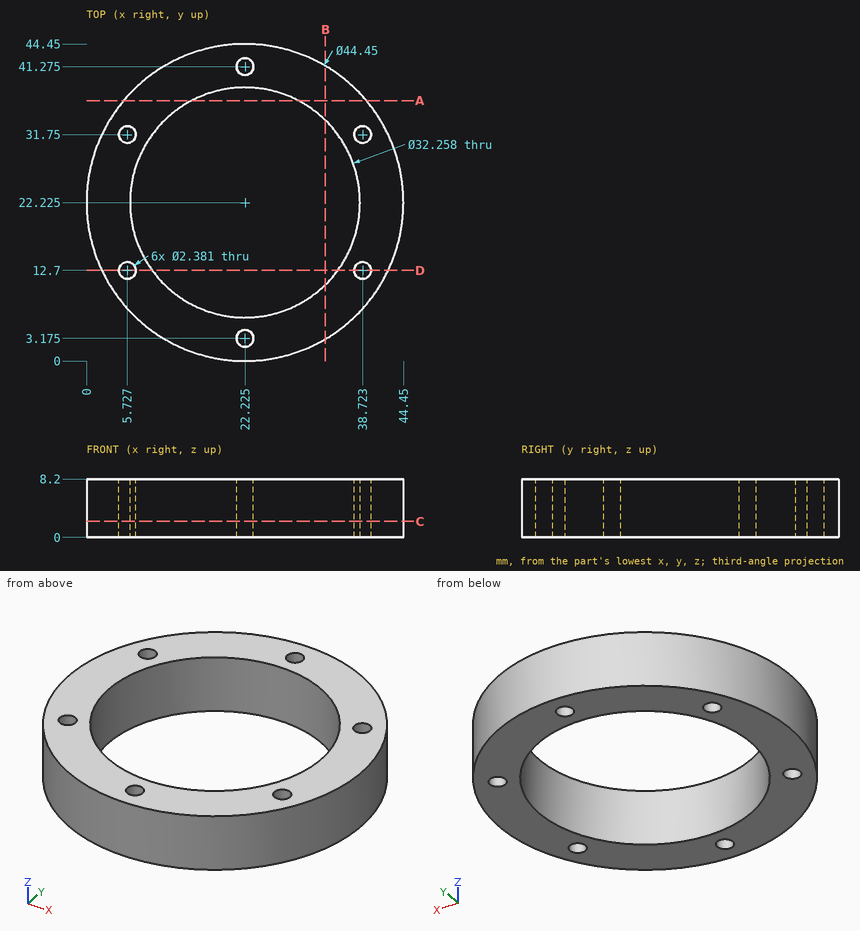
Study the drawing (mm; zero at the part's minimum x, y, z) and answer. Round coordinates to 2 decimals unless told otherwise and drop trailing zeros. Write each loop counter-clockwise with the first axis right and the second up, starting at its lowest first coordinate (ties: lowest second). Pieces come first, ordered by that corner, then holes. Notation, with made-up numbers: (35, 3.5) -> (89, 3.5) arc R25 ccw to (89, 30.5) -> close; hole circle Ø6 at (-32.5, 49.25). An arc over 180 degrees is marked (long way). Write each question's results on one line, items separated by ' | '.
Item 1: A cutting plane is placed at B-B, the plane x = 33.5. Determine the outline of the cut face in (y, z).
Result set:
outline: (3.07, 0) -> (10.69, 0) -> (10.69, 8.2) -> (3.07, 8.2) -> close; (33.76, 0) -> (41.38, 0) -> (41.38, 8.2) -> (33.76, 8.2) -> close
Item 2: Find the intervals of material crossed by line 1 along Y through (x, z) = (39, 6.75) (1 decimal); line 2 along X through (y, z) = (12.7, 5.5) (1 decimal); line 3 along Y through (x, z) = (18.5, 1.5) (1 decimal), in increasing order. Write a range as [from, to].
Result set:
line 1: [7.6, 11.5], [13.9, 30.6], [32.9, 36.8] | line 2: [2.1, 4.5], [6.9, 9.2], [35.2, 37.5], [39.9, 42.3] | line 3: [0.3, 6.5], [37.9, 44.1]
Item 3: A cutting plane is placed at D-D, the plane y = 12.7. Determine the outline of the cut face in (x, z) (1 decimal).
Result set:
outline: (2.1, 0) -> (4.5, 0) -> (4.5, 8.2) -> (2.1, 8.2) -> close; (6.9, 0) -> (9.2, 0) -> (9.2, 8.2) -> (6.9, 8.2) -> close; (35.2, 0) -> (37.5, 0) -> (37.5, 8.2) -> (35.2, 8.2) -> close; (39.9, 0) -> (42.3, 0) -> (42.3, 8.2) -> (39.9, 8.2) -> close
Item 4: Flat-ended cylindrical pins translate along their axes: P1, Ø1.4, axis at x = 5.73, y = 31.75, coming from the +Z side; P2, Ø2, axis at y = 30, z = 4.5, coming from the -X side; P3, Ø4, axis at x = 22, z = 3.5, coming from the +Y side; P4, Ø3, axis at x = 11, z = 2.5, coming from the -Y side. Find the tip coordinate at first contact, or state that the pin passes through.
Result set:
P1: through | P2: x = 1.06 | P3: y = 44.45 | P4: y = 2.24
Item 5: A cutting plane is placed at C-C, the plane z = 2.25. Count the separate pieces of the cut face and the enclosed holes in it, plus the area to 3 significant figures.
Result set:
separate pieces: 1 | enclosed holes: 7 | area: 708 mm^2
Item 6: A cutting plane is placed at A-A, the plane y = 36.5. Determine the outline of the cut face in (x, z).
Result set:
outline: (5.19, 0) -> (14.72, 0) -> (14.72, 8.2) -> (5.19, 8.2) -> close; (29.73, 0) -> (39.26, 0) -> (39.26, 8.2) -> (29.73, 8.2) -> close
